```python
from build123d import *

# Parameters (mm, degrees)
SKETCH1_R           = 31
BOSS_EXTRUDE1_DEPTH = 4
SKETCH3_R           = 6.5
BOSS_EXTRUDE2_DEPTH = 32
BOSS_EXTRUDE2_TAPER = 5
SKETCH4_R           = 2
CUT_EXTRUDE1_DEPTH  = 85.297093663
SKETCH5_W           = 0.5
SKETCH5_H           = 0.5
CUT_EXTRUDE2_DEPTH  = 0.5


with BuildPart() as part:
    # Sketch1 → Boss-Extrude1 (new, symmetric)
    with BuildSketch(Plane.XY):
        Circle(SKETCH1_R)
    extrude(amount=BOSS_EXTRUDE1_DEPTH, both=True)

    # Sketch3 → Boss-Extrude2 (add)
    with BuildSketch(Plane.XY.offset(4)):
        Circle(SKETCH3_R)
    boss_extrude2 = extrude(amount=BOSS_EXTRUDE2_DEPTH, taper=BOSS_EXTRUDE2_TAPER)

    # Mirror1: Boss-Extrude2 across plane
    add(boss_extrude2.mirror(Plane.XY))

    # Sketch4 → Cut-Extrude1 (cut, through all)
    with BuildSketch(Plane.XY.offset(36)):
        Circle(SKETCH4_R)
    extrude(amount=-CUT_EXTRUDE1_DEPTH, mode=Mode.SUBTRACT)

    # Sketch5 → Cut-Extrude2 (cut)
    with BuildSketch(Plane.XY.offset(4)):
        with Locations((20, 0)):
            Rectangle(SKETCH5_W, SKETCH5_H)
    extrude(amount=-CUT_EXTRUDE2_DEPTH, mode=Mode.SUBTRACT)


solid = part.part
```
Input: part model. Units: mm. Frame: model coordinates. Coordinates: 2 decimals unless noted, no trailing zeros. Loops run counter-clockwise (first coordinate to the right, second up) from the corner with the lowest first, then second, coordinate; pieces in that order, holes last. Notation, with made-up numbers: M 26.25,-16 L 60.25,-16 A18 cw 60.25,6 Z; hole C -12,23.25 d4. An arc over 180 degrees is marked long. One line per item, written item: value.
(1) Pin query (flat end, axial travel): pin 1 (1.5 mm diameter, centred on x = -18, y = 22, fed in from +Z); pin 2 (4 mm diameter, centred on y = 3, z = -25.5, fed in from -X); pin 3 (10 mm diameter, centred on x = -11.5, y = 7, fed in from -Z); pin 4 (6 mm diameter, centred on y = 0.5, z = -2.5, fed in from +X). Return the tip coordinate at first contact, or that it passes through.
Filled in:
pin 1: z = 4
pin 2: x = -4.54
pin 3: z = -4
pin 4: x = 31
(2) Section C-C (y = -13). Output: boundary loops of the cut face in (x, z), and give its area (3 significant figures).
Filled in:
outline: M -28.14,-4 L 28.14,-4 L 28.14,4 L -28.14,4 Z
area: 450 mm^2
(3) Pull-direction query (Y, two-part tool) for faces 1 (the cylindrical face through (0, -2, 1)), 2 (the conical face through (4.846, 1.526, -20.224)), 3 (the flat face through (2, -2, -36)); classes: +Y half, -Y half, draft (parallel to the pull), parting line (faces both ways), or undercut.
Filled in:
face 1: undercut
face 2: parting line
face 3: draft
(4) Line query: line 1 along Z through (x, y) = (0, -16); line 2 along Y through (x, z) = (0, -9.5); line 3 along Y through (x, z) = (0, 4.5). Output: solid intervals per line, ascending. Write a range as from..to.
Filled in:
line 1: -4..4
line 2: -6.02..-2, 2..6.02
line 3: -6.46..-2, 2..6.46
(5) Section D-D (x = -11). Output: boundary loops of the cut face in (y, z).
Filled in:
outline: M -28.98,-4 L 28.98,-4 L 28.98,4 L -28.98,4 Z
(6) Section B-B (z = -26). Output: boundary loops of the cut face in (x, y).
Filled in:
outline: C 0,0 d9.15; hole C 0,0 d4
(7) Section A-A (x = 0). Output: boundary loops of the cut face in (y, z).
Filled in:
outline: M -31,-4 L -6.5,-4 L -3.7,-36 L -2,-36 L -2,36 L -3.7,36 L -6.5,4 L -31,4 Z; M 2,-36 L 3.7,-36 L 6.5,-4 L 31,-4 L 31,4 L 6.5,4 L 3.7,36 L 2,36 Z
